Autodesk Inventor part; units mm, degrees
ref_plane "YZ Plane" through (0, 0, 0) normal (1, 0, 0) x (0, 1, 0)
ref_plane "XZ Plane" through (0, 0, 0) normal (0, 1, 0) x (-1, 0, 0)
ref_plane "XY Plane" through (0, 0, 0) normal (0, 0, 1) x (1, 0, 0)
sketch "Sketch1" plane through (0, 0, 0) normal (0, 0, 1) x (1, 0, 0)
  circle A0 centre (0, 0) radius 2.5
  dimension "d0" = 5
extrude "Extrusion1" add sketch "Sketch1" along normal blind 50
sketch "Sketch2" plane through (0, 0, 0) normal (0, 0, -1) x (-1, 0, 0)
  circle A0 centre (0, 0) radius 2.5
  circle A1 centre (0, 0) radius 4.25
  dimension "d3" = 8.5
extrude "Extrusion2" add sketch "Sketch2" along normal blind 5 contours A0 | A1
sketch "Sketch3" plane through (0, 0, -5) normal (0, 0, -1) x (-1, 0, 0)
  circle A0 centre (0, 0) radius 4.25
  line L0 (-1.1547, 2) -> (1.1547, 2)
  line L1 (1.1547, 2) -> (2.3094, 0)
  line L2 (2.3094, 0) -> (1.1547, -2)
  line L3 (1.1547, -2) -> (-1.1547, -2)
  line L4 (-1.1547, -2) -> (-2.3094, 0)
  line L5 (-2.3094, 0) -> (-1.1547, 2)
  dimension "d6" = 4
extrude "Extrusion3" cut sketch "Sketch3" against normal blind 2.5 contours L0 L1 L2 L3 L4 L5
thread "Thread1"
chamfer "Chamfer1" distance 0.508 angle 45 1 edges at (-2.5, 0, 50)
fillet "Fillet1" radius 0.508 2 edges at (4.25, 0, -5) (4.25, 0, 0)
properties part number "m5 x50" material "Steel"
For this review, take the finished solid that the model builds, in its own axes (mm). A direction names the side the tool comes from. Round coordinates to 2 decimals unless told otherwise and drop trailing zeros. Order: outer loops, then holes, each group sorted by start corner. A loop starts at its lowest first (then second) coordinate and runs counter-clockwise, first axis right, second up. Notation, with made-up numbers: M -21,-11 L 16,-11 A4 cw 16,-6 Z; hole C 54.25,33 d1. An arc over 180 degrees is marked long. Use a Markdown table: item, result. Add a question column.
Item 1: Insertion check: pin 1 (2 mm diameter, centred on x = -0.5, y = 1.5, fed in from -Z); pin 2 (2 mm diameter, centred on y = -0.5, z = 37, fed in from -X); pin 3 (4 mm diameter, centred on x = 3, z = 32, fed in from -Y); pin 4 (1.2 mm diameter, centred on x = 0.5, y = -0.5, fed in from -Z). Each pin has a flat end and moves straight along its axis. Give the tip position at first contact, or say it passes through.
Item 2: To check wall thickness, follow line 1 along Y through (x, z) = (-1.5, 19); line 2 along Z through (x, y) = (2.75, 0.25). State the ranges of each line that lie inside material, in increasing order.
Item 3: Add section B-B, the plane z = 34.5. Give the boundary of the cut face in (x, y), then the cut area to 3 significant figures.
Item 4: Add section A-A, the plane x = 0. Give the boundary of the cut face in (y, z).
Item 5: Mouldability with a two-part tool opening along Y and no side actions: class faces 1 (the cylindrical face through (-0.54, 2.44, 24.4)), 2 (the flat face through (0, 0, 50)), 3 (the flat face through (-1.724, 1.014, -3.768)) as released by +Y, released by -Y, zero draft, split by the parting line, or undercut.
Item 6: Tool access review of faces 4 (the flat face through (0, 3, 0)), 5 (the cylindrical face through (-2.285, -3.584, -2.472)), 6 (the flat face through (-1.74, -0.99, -3.77)): name each direction out of +Z, -Z, +X, -X, +Y, -Y from which nothing blocks a thin tool from reaching the whole face with its end or side.
Geometry results:
| question | item | result |
|---|---|---|
| 1 | pin 1 | stops at z = -5 |
| 1 | pin 2 | stops at x = -2.5 |
| 1 | pin 3 | stops at y = -2.29 |
| 1 | pin 4 | stops at z = -2.5 |
| 2 | line 1 | y = -2 to 2 |
| 2 | line 2 | z = -5 to 0 |
| 3 | outline | C 0,0 d5 |
| 3 | area | 19.6 mm² |
| 4 | outline | M -4.25,-4.49 A0.51 ccw -3.74,-5 L -2,-5 L -2,-2.5 L 2,-2.5 L 2,-5 L 3.74,-5 A0.51 ccw 4.25,-4.49 L 4.25,-0.51 A0.51 ccw 3.74,0 L 2.5,0 L 2.5,49.49 L 1.99,50 L -1.99,50 L -2.5,49.49 L -2.5,0 L -3.74,0 A0.51 ccw -4.25,-0.51 Z |
| 5 | face 1 | split by the parting line |
| 5 | face 2 | zero draft |
| 5 | face 3 | undercut |
| 6 | face 4 | +Z |
| 6 | face 5 | +Z, -Z |
| 6 | face 6 | -Z |
